```python
from build123d import *

# Parameters (mm, degrees)
BOSS_EXTRUDE1_DEPTH     = 6.35
CUT_EXTRUDE3_DEPTH      = 602.409033022
CUT_EXTRUDE3_DEPTH_BACK = 602.409033022
SKETCH10_R              = 5.0000027
SKETCH2_R               = 2.778125
CUT_EXTRUDE4_DEPTH      = 602.409033022


with BuildPart() as part:
    # Sketch1 → Boss-Extrude1 (new body)
    with BuildSketch(Plane(origin=(0, 0, 0), x_dir=(1, 0, 0), z_dir=(0, 1, 0))):
        Polygon((0, 0), (0, 177.8), (-114.3, 177.8), (-114.3, 222.25), (-558.8, 222.25), (-558.8, 0), align=None)
    extrude(amount=BOSS_EXTRUDE1_DEPTH)

    # Sketch10 → Cut-Extrude3 (cut, two sides: drawn at the far end of the back side and taken through both)
    with BuildSketch(Plane(origin=(0, 6.35, 0), x_dir=(1, 0, 0), z_dir=(0, 1, 0)).offset(-CUT_EXTRUDE3_DEPTH_BACK)):
        with Locations(Location((-481.076, 40.132, 0), (0, 0, 270))):
            Circle(SKETCH10_R)
        with Locations(Location((-356.108, 40.132, 0), (0, 0, 270))):
            Circle(SKETCH10_R)
        with Locations(Location((-231.14, 40.132, 0), (0, 0, 270))):
            Circle(SKETCH10_R)
        with Locations(Location((-356.108, 140.208, 0), (0, 0, 270))):
            Circle(SKETCH10_R)
        with Locations(Location((-231.14, 140.208, 0), (0, 0, 270))):
            Circle(SKETCH10_R)
        with Locations(Location((-481.076, 140.208, 0), (0, 0, 270))):
            Circle(SKETCH10_R)
    extrude(amount=CUT_EXTRUDE3_DEPTH + CUT_EXTRUDE3_DEPTH_BACK, mode=Mode.SUBTRACT)

    # Sketch2 → Cut-Extrude4 (cut, through all)
    with BuildSketch(Plane.XZ):
        with Locations(Location((-52.1589, -86.783333333, 0), (0, 0, 270))):
            Circle(SKETCH2_R)
        with Locations(Location((-52.1589, -65.616666667, 0), (0, 0, 270))):
            Circle(SKETCH2_R)
        with Locations(Location((-469.142233333, -185.187166667, 0), (0, 0, 270))):
            Circle(SKETCH2_R)
        with Locations(Location((-486.075566667, -168.253833333, 0), (0, 0, 270))):
            Circle(SKETCH2_R)
    extrude(amount=-CUT_EXTRUDE4_DEPTH, mode=Mode.SUBTRACT)


solid = part.part
```
Check sheet for the modelled part. Datum: model origin and axes. Units: mm. Give positions to 0.01 mm unless a question says otherwise; leave off trailing zeros. Write each loop counter-clockwise with the first axis right and the second up, starting at its lowest first coordinate (ties: lowest second). Pieces come first, ordered by that corner, then holes.
Item 1: Cross-section at A-A (x = -231.14). Enter the section's corners in (y, z).
Item 2: Gauge pin test, flat end, axial feed: pin 1 (1.9 mm diameter, centred on y = 3, z = -196.5, fed in from +X). Record the tip position at first contact, or that the pin passes through.
Item 3: Scan lines: L1, parallel to Z at x = -231.14, y = 3.5; L2, parallel to Z at x = -36, y = 3; L3, parallel to X at y = 5.5, z = -201. Record each from-to range of solid material in increasing order.
Item 4: Draft check along Z on faces 1 (the face through (-485.5, 3.1, -37.8)), 2 (the face through (-283, 0, -113)), 3 (the face through (-236.02, 3.13, -141.29)). Enter one of: released by +Z, released by -Z, zero draft, split by the parting line, or undercut.
Item 5: Cross-section at B-B (y = 3). Count the separate pieces of the cut face and the enclosed holes in it, and give its area (3 significant figures).
Report:
1. outline: (0, -222.25) - (6.35, -222.25) - (6.35, -145.21) - (0, -145.21) - close; (0, -135.21) - (6.35, -135.21) - (6.35, -45.13) - (0, -45.13) - close; (0, -35.13) - (6.35, -35.13) - (6.35, 0) - (0, 0) - close
2. pin 1: stops at x = -114.3
3. L1: z = -222.25 to -145.21, -135.21 to -45.13, -35.13 to 0
3. L2: z = -177.8 to 0
3. L3: x = -558.8 to -114.3
4. face 1: undercut
4. face 2: zero draft
4. face 3: undercut
5. separate pieces: 1
5. enclosed holes: 10
5. area: 119,000 mm2
